Geometry: final body of the model. Coordinates: model frame, mm. A direction names the side the tool comes from. Round coordinates to 2 decimals unless told otherwise and drop trailing zeros. Order: outer loops, then holes, each group sorted by start corner. A loop starts at its lowest first (then second) coordinate and runs counter-clockwise, first axis right, second up. Notation, with made-up numbers: (12, 38.5) - (52, 38.5) arc R31 cw to (52, 68.5) - close; hole circle Ø4 at (32, 62). An arc over 180 degrees is marked (long way). Put each result on its own line as item: value. Start each with the question number.
(1) Material intervals for L1, parallel to X at y = 10, z = 0.3; L2, parallel to X at y = -23, z = 1.6; L3, parallel to Y at x = -12, z = 1.35, sorted ascending. Write a range as [from, to].
(2) Pin query (flat end, axial travel): P1, Ø1.5, axis at x = -11.5, y = -22, coming from the -Z side; P2, Ø0.6, axis at x = 18, z = 1, coming from the -Y side. Return the tip coordinate at first contact, or that it passes through.
(3) Pull-direction query (Y, two-part tool) for faces 1 (the face through (10.13, -37, 0.99)), 2 (the face through (8.64, 39.92, 0.99)), 3 (the face through (-19.175, -17.972, 1.014)), 4 (the face through (23, -33, 1)); classes: released by +Y, released by -Y, zero draft, split by the parting line, or undercut.
(4) Section D-D (z = 1.6). Count the separate pieces of the cut face and the enclosed holes in it, and give its area (3 significant figures).
(5) Access query for faces 5 (the face through (19.175, 25.972, 1.014)), 6 (the face through (18, -33.85, 1)), 7 (the face through (-19.166, 25.937, 1.014)), 8 (the face through (17.31, -38.85, 0.99)). Directions: +Z, -Z, +X, -X, +Y, -Y. A direction counts if a zero-diameter tool reaches every point of the face in a straight line with its end or side. Return the directions, or none.
(6) Section C-C (x = -18). Output: boundary loops of the cut face in (y, z), and give its area (3 significant figures).
(7) Section B-B (x = 11). Output: boundary loops of the cut face in (y, z).
(8) Section A-A (y = -32.6). Output: boundary loops of the cut face in (x, z).
from build123d import *

# Parameters (mm, degrees)
F0_R      = 1.6
F1_DEPTH  = 2
F2_W      = 6
F2_H      = 4
F2_R      = 1.6
F2_R_2    = 3.5
F2_R_3    = 8
F3_DEPTH  = 2.001
F5_DEPTH  = 2.001
F6_R      = 5
F7_R      = 1
F8_R      = 2
F10_DEPTH = 2.0010001


with BuildPart() as f1:
    # F0 (on Top) → F1 (new body)
    with BuildSketch(Plane.XY):
        with BuildLine():
            ThreePointArc((-22.4, 38.8525709713), (-22.8439088915, 38.1988819549), (-23, 37.4242852856))
            Line((-23, 37.4242852856), (-23, -39.0255160858))
            ThreePointArc((-23, -39.0255160858), (-21.8744746322, -40.8242084212), (-19.7647058824, -40.5984269042))
            ThreePointArc((-19.7647058824, -40.5984269042), (-17.3419245059, -38.8715499716), (-14.7692307692, -37.3771536131))
            ThreePointArc((-14.7692307692, -37.3771536131), (-8.88675287, -37.5707723251), (-6, -42.6998748107))
            Line((-6, -42.6998748107), (-6, -45))
            ThreePointArc((-6, -45), (0, -51), (6, -45))
            Line((6, -45), (6, -42.6998748107))
            ThreePointArc((6, -42.6998748107), (8.88675287, -37.5707723251), (14.7692307692, -37.3771536131))
            ThreePointArc((14.7692307692, -37.3771536131), (17.3419245059, -38.8715499716), (19.7647058824, -40.5984269042))
            ThreePointArc((19.7647058824, -40.5984269042), (21.8744746322, -40.8242084212), (23, -39.0255160858))
            Line((23, -39.0255160858), (23, 37.4242852856))
            ThreePointArc((23, 37.4242852856), (22.8439088915, 38.1988819549), (22.4, 38.8525709713))
            ThreePointArc((22.4, 38.8525709713), (17.5812540395, 42.7376047244), (12.1046910387, 45.6222290663))
            ThreePointArc((12.1046910387, 45.6222290663), (10.3819905013, 45.5219936492), (9.3785323428, 44.118136105))
            Line((9.3785323428, 44.118136105), (7.8784620241, 35.6108145787))
            ThreePointArc((7.8784620241, 35.6108145787), (0, 29), (-7.8784620241, 35.6108145787))
            Line((-7.8784620241, 35.6108145787), (-9.3785323428, 44.118136105))
            ThreePointArc((-9.3785323428, 44.118136105), (-10.3819905013, 45.5219936492), (-12.1046910387, 45.6222290663))
            ThreePointArc((-12.1046910387, 45.6222290663), (-17.5812540395, 42.7376047244), (-22.4, 38.8525709713))
        make_face()
        with Locations((-18, -28)):
            Circle(F0_R, mode=Mode.SUBTRACT)
        with Locations((18, -28)):
            Circle(F0_R, mode=Mode.SUBTRACT)
        with Locations((-18, 37)):
            Circle(F0_R, mode=Mode.SUBTRACT)
        with Locations((18, 37)):
            Circle(F0_R, mode=Mode.SUBTRACT)
    extrude(amount=F1_DEPTH)

    # F2 (on face) → F3 (cut, through all)
    with BuildSketch(Plane.XY.offset(2)):
        with Locations((-7, -43)):
            Rectangle(F2_W, F2_H)
        with Locations((7, -43)):
            Rectangle(F2_W, F2_H)
        with BuildLine():
            Line((-5, -34), (-5, -31.5))
            ThreePointArc((-5, -31.5), (-6.25, -30.25), (-7.5, -31.5))
            Line((-7.5, -31.5), (-7.5, -34))
            ThreePointArc((-7.5, -34), (-6.25, -35.25), (-5, -34))
        make_face()
        with BuildLine():
            ThreePointArc((7.5, -31.5), (6.25, -30.25), (5, -31.5))
            Line((5, -31.5), (5, -34))
            ThreePointArc((5, -34), (6.25, -35.25), (7.5, -34))
            Line((7.5, -34), (7.5, -31.5))
        make_face()
        with Locations((-11, -11.5)):
            Circle(F2_R)
        with Locations((11, -11.5)):
            Circle(F2_R)
        with Locations((0, -25)):
            Circle(F2_R_2)
        with Locations((0, -56)):
            Circle(F2_R_3)
    extrude(amount=-F3_DEPTH, mode=Mode.SUBTRACT)

    # F4 (on face) → F5 (cut, through all)
    with BuildSketch(Plane.XY.offset(2)):
        with BuildLine():
            Line((-19, -16.6602540378), (-19, 24.6602540378))
            ThreePointArc((-19, 24.6602540378), (-19.1703708686, 25.9543492634), (-19.6698729811, 27.1602540378))
            Line((-19.6698729811, 27.1602540378), (-23, 32.9282032303))
            Line((-23, 32.9282032303), (-23, -24.9282032303))
            Line((-23, -24.9282032303), (-19.6698729811, -19.1602540378))
            ThreePointArc((-19.6698729811, -19.1602540378), (-19.1703708686, -17.9543492634), (-19, -16.6602540378))
        make_face()
        with BuildLine():
            ThreePointArc((19.6698729811, 27.1602540378), (19.1703708686, 25.9543492634), (19, 24.6602540378))
            Line((19, 24.6602540378), (19, -16.6602540378))
            ThreePointArc((19, -16.6602540378), (19.1703708686, -17.9543492634), (19.6698729811, -19.1602540378))
            Line((19.6698729811, -19.1602540378), (23, -24.9282032303))
            Line((23, -24.9282032303), (23, 32.9282032303))
            Line((23, 32.9282032303), (19.6698729811, 27.1602540378))
        make_face()
    extrude(amount=-F5_DEPTH, mode=Mode.SUBTRACT)

    # F6
    f6_edges = [f1.edges().sort_by_distance(p)[0] for p in [
        (-23, 32.928203, 1),
        (23, 32.928203, 1),
        (23, -24.928203, 1),
        (-23, -24.928203, 1),
    ]]
    fillet(f6_edges, radius=F6_R)

    # F7
    f7_edges = [f1.edges().sort_by_distance(p)[0] for p in [
        (-4, -41, 1),
        (-4, -45, 1),
        (4, -41, 1),
        (4, -45, 1),
    ]]
    fillet(f7_edges, radius=F7_R)

    # F8
    f8_edges = [f1.edges().sort_by_distance(p)[0] for p in [
        (-6.245834, -41, 1),
        (6.245834, -41, 1),
        (-6, -45, 1),
        (6, -45, 1),
    ]]
    fillet(f8_edges, radius=F8_R)

    # F9 (on face) → F10 (cut, through all)
    with BuildSketch(Plane.XY.offset(2)):
        with BuildLine():
            ThreePointArc((-16.75, -33.85), (-15.5, -32.6), (-16.75, -31.35))
            Line((-16.75, -31.35), (-19.25, -31.35))
            ThreePointArc((-19.25, -31.35), (-20.5, -32.6), (-19.25, -33.85))
            Line((-19.25, -33.85), (-16.75, -33.85))
        make_face()
        with BuildLine():
            Line((19.25, -31.35), (16.75, -31.35))
            ThreePointArc((16.75, -31.35), (15.5, -32.6), (16.75, -33.85))
            Line((16.75, -33.85), (19.25, -33.85))
            ThreePointArc((19.25, -33.85), (20.5, -32.6), (19.25, -31.35))
        make_face()
    extrude(amount=-F10_DEPTH, mode=Mode.SUBTRACT)


solid = f1.part
Checks:
1. L1: x = [-19, 19]
1. L2: x = [-21.89, -2.87], [2.87, 21.89]
1. L3: y = [-36.7, -12.75], [-10.25, 45.66]
2. P1: stops at z = 0
2. P2: stops at y = -39.51
3. face 1: released by -Y
3. face 2: released by +Y
3. face 3: undercut
3. face 4: zero draft
4. separate pieces: 1
4. enclosed holes: 11
4. area: 3,110 mm²
5. face 5: +Z, -Z, +X
5. face 6: +Z, -Z
5. face 7: +Z, -Z, -X
5. face 8: +Z, -Z, -Y
6. outline: (-39.31, 0) - (-33.85, 0) - (-33.85, 2) - (-39.31, 2) - close; (-31.35, 0) - (-29.6, 0) - (-29.6, 2) - (-31.35, 2) - close; (-26.4, 0) - (35.4, 0) - (35.4, 2) - (-26.4, 2) - close; (38.6, 0) - (42.46, 0) - (42.46, 2) - (38.6, 2) - close
6. area: 146 mm²
7. outline: (-36.78, 0) - (-13.1, 0) - (-13.1, 2) - (-36.78, 2) - close; (-9.9, 0) - (45.74, 0) - (45.74, 2) - (-9.9, 2) - close
8. outline: (-23, 0) - (-20.5, 0) - (-20.5, 2) - (-23, 2) - close; (-15.5, 0) - (-7.5, 0) - (-7.5, 2) - (-15.5, 2) - close; (-5, 0) - (5, 0) - (5, 2) - (-5, 2) - close; (7.5, 0) - (15.5, 0) - (15.5, 2) - (7.5, 2) - close; (20.5, 0) - (23, 0) - (23, 2) - (20.5, 2) - close
